```python
from build123d import *

# Parameters (mm, degrees)
F0_W        = 100
F0_H        = 50
F1_DEPTH    = 50
F2_T        = -2.5
F3_W        = 50
F3_H        = 70.2898527046
F4_DEPTH    = 25
F5_R        = 5
F6_DEPTH    = 50
F7_T1_DEPTH = 75
F7_T3_DEPTH = 75
F8_T1_DEPTH = 2.5
F8_T3_DEPTH = 2.5
F8_T5_DEPTH = 75
F9_T1_DEPTH = 75
F9_T3_DEPTH = 75
F10_R       = 11.25
F11_DEPTH   = 100


# Not quite as in the source:
# - a fillet or chamfer that OpenCascade refuses, or shapes differently, is made with other operations: its cross-section is extruded or revolved along the edge and cut away or added


with BuildPart() as f1:
    # F0 (on Top) → F1 (new body)
    with BuildSketch(Plane.XY):
        with Locations((50, 25)):
            Rectangle(F0_W, F0_H)
    extrude(amount=F1_DEPTH)

    # F2
    f2_openings = [f1.faces().sort_by_distance(p)[0] for p in [
        (50, 25, 0),
    ]]
    offset(amount=F2_T, openings=f2_openings)

    # F3 (on face) → F4 (cut)
    with BuildSketch(Plane.XY.offset(50)):
        with Locations((50, 24.9999999069)):
            Rectangle(F3_W, F3_H)
    extrude(amount=-F4_DEPTH, mode=Mode.SUBTRACT)

    # F5 (on face) → F6 (cut)
    with BuildSketch(Plane.XZ):
        with Locations((12.5, 12.5)):
            Circle(F5_R)
        with Locations((87.5, 12.5)):
            Circle(F5_R)
    extrude(amount=-F6_DEPTH, mode=Mode.SUBTRACT)

    # F7: fillet of radius 5 on 4 edges, made by hand

    # F7_s2 → F7_t1 (cut)
    with BuildSketch(Plane.XZ.offset(-62.5)):
        with BuildLine():
            ThreePointArc((0, 45), (1.4644660941, 48.5355339059), (5, 50))
            Line((5, 50), (0, 50))
            Line((0, 50), (0, 45))
        make_face()
        with BuildLine():
            ThreePointArc((0, 5), (1.4644660941, 1.4644660941), (5, 0))
            Line((5, 0), (0, 0))
            Line((0, 0), (0, 5))
        make_face()
    extrude(amount=F7_T1_DEPTH, mode=Mode.SUBTRACT)

    # F7_s4 → F7_t3 (cut)
    with BuildSketch(Plane.XY.offset(-12.5)):
        with BuildLine():
            ThreePointArc((0, 5), (1.4644660941, 1.4644660941), (5, 0))
            Line((5, 0), (0, 0))
            Line((0, 0), (0, 5))
        make_face()
        with BuildLine():
            ThreePointArc((0, 45), (1.4644660941, 48.5355339059), (5, 50))
            Line((5, 50), (0, 50))
            Line((0, 50), (0, 45))
        make_face()
    extrude(amount=F7_T3_DEPTH, mode=Mode.SUBTRACT)

    # F8: fillet of radius 5 on 6 edges, made by hand

    # F8_s2 → F8_t1 (join)
    with BuildSketch(Plane.XZ.offset(-2.5)):
        with BuildLine():
            ThreePointArc((25, 30), (26.4644660941, 26.4644660941), (30, 25))
            Line((30, 25), (25, 25))
            Line((25, 25), (25, 30))
        make_face()
        with BuildLine():
            ThreePointArc((75, 30), (73.5355339059, 26.4644660941), (70, 25))
            Line((70, 25), (75, 25))
            Line((75, 25), (75, 30))
        make_face()
    extrude(amount=F8_T1_DEPTH)

    # F8_s4 → F8_t3 (join)
    with BuildSketch(Plane.XZ.offset(-50)):
        with BuildLine():
            ThreePointArc((25, 30), (26.4644660941, 26.4644660941), (30, 25))
            Line((30, 25), (25, 25))
            Line((25, 25), (25, 30))
        make_face()
        with BuildLine():
            ThreePointArc((70, 25), (73.5355339059, 26.4644660941), (75, 30))
            Line((75, 30), (75, 25))
            Line((75, 25), (70, 25))
        make_face()
    extrude(amount=F8_T3_DEPTH)

    # F8_s6 → F8_t5 (cut)
    with BuildSketch(Plane.XZ.offset(-62.5)):
        with BuildLine():
            ThreePointArc((20, 50), (23.5355339059, 48.5355339059), (25, 45))
            Line((25, 45), (25, 50))
            Line((25, 50), (20, 50))
        make_face()
        with BuildLine():
            ThreePointArc((75, 45), (76.4644660941, 48.5355339059), (80, 50))
            Line((80, 50), (75, 50))
            Line((75, 50), (75, 45))
        make_face()
    extrude(amount=F8_T5_DEPTH, mode=Mode.SUBTRACT)

    # F9: fillet of radius 5 on 4 edges, made by hand

    # F9_s2 → F9_t1 (cut)
    with BuildSketch(Plane.XZ.offset(-62.5)):
        with BuildLine():
            ThreePointArc((100, 45), (98.5355339059, 48.5355339059), (95, 50))
            Line((95, 50), (100, 50))
            Line((100, 50), (100, 45))
        make_face()
        with BuildLine():
            ThreePointArc((95, 0), (98.5355339059, 1.4644660941), (100, 5))
            Line((100, 5), (100, 0))
            Line((100, 0), (95, 0))
        make_face()
    extrude(amount=F9_T1_DEPTH, mode=Mode.SUBTRACT)

    # F9_s4 → F9_t3 (cut)
    with BuildSketch(Plane.XY.offset(-12.5)):
        with BuildLine():
            ThreePointArc((95, 0), (98.5355339059, 1.4644660941), (100, 5))
            Line((100, 5), (100, 0))
            Line((100, 0), (95, 0))
        make_face()
        with BuildLine():
            ThreePointArc((95, 50), (98.5355339059, 48.5355339059), (100, 45))
            Line((100, 45), (100, 50))
            Line((100, 50), (95, 50))
        make_face()
    extrude(amount=F9_T3_DEPTH, mode=Mode.SUBTRACT)

    # F10 (on face) → F11 (cut)
    with BuildSketch(Plane.YZ.offset(100)):
        with Locations((25, 25.6698729811)):
            Circle(F10_R)
    extrude(amount=-F11_DEPTH, mode=Mode.SUBTRACT)


solid = f1.part
```
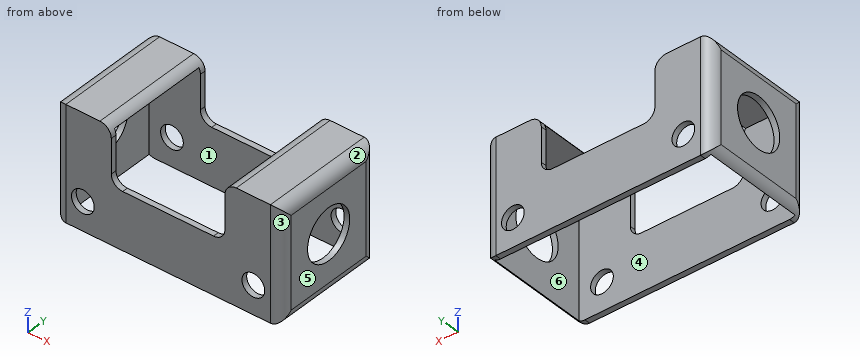
Input: part model. Units: mm. Frame: model coordinates. Face numbers are marked on the shaded views. A direction names the side the tool comes from. Round coordinates to 2 decimals unless told otherwise and drop trailing zeros. Write each loop counter-clockwise with the first axis right and the second up, starting at its lowest first coordinate (ties: lowest second). Pieces come first, ordered by that corner, then holes. Notation, with made-up numbers: (22, 86.5) - (76, 86.5) arc R21 cw to (76, 111.5) - close; hole circle Ø6 at (21, -26.5). An arc over 180 degrees is marked (long way). Write item = value, one per line.
(1) Section query D-D on y = 25. Output: boundary loops of the cut face in (x, z).
Geometry check:
outline = (0, 5) arc R5 ccw to (2.5, 0.67) - (2.5, 14.42) - (0, 14.42) - close; (0, 36.92) - (2.5, 36.92) - (2.5, 47.5) - (24.33, 47.5) arc R5 ccw to (20, 50) - (5, 50) arc R5 ccw to (0, 45) - close; (75.67, 47.5) - (97.5, 47.5) - (97.5, 36.92) - (100, 36.92) - (100, 45) arc R5 ccw to (95, 50) - (80, 50) arc R5 ccw to start; (97.5, 0.67) arc R5 ccw to (100, 5) - (100, 14.42) - (97.5, 14.42) - close
(2) Section query A-A on x = 62. Output: boundary loops of the cut face in (y, z).
Geometry check:
outline = (0, 0) - (2.5, 0) - (2.5, 25) - (0, 25) - close; (47.5, 0) - (50, 0) - (50, 25) - (47.5, 25) - close
(3) Section query B-B on y = 8. Output: boundary loops of the cut face in (x, z), then the cut area to 3 significant figures.
Geometry check:
outline = (0, 5) arc R5 ccw to (2.5, 0.67) - (2.5, 47.5) - (24.33, 47.5) arc R5 ccw to (20, 50) - (5, 50) arc R5 ccw to (0, 45) - close; (75.67, 47.5) - (97.5, 47.5) - (97.5, 0.67) arc R5 ccw to (100, 5) - (100, 45) arc R5 ccw to (95, 50) - (80, 50) arc R5 ccw to start
area = 332 mm^2
(4) Material intervals for probe 1 along Y at (x, z) = (95, 22.5); probe 2 along X at (y, z) = (37.5, 29.5); probe 3 along Z at (x, y) = (12.5, 1.9), sorted ascending.
Geometry check:
probe_1 = 0 to 2.5, 47.5 to 50
probe_2 = 0 to 2.5, 97.5 to 100
probe_3 = 0 to 7.5, 17.5 to 50
(5) Access query for the marked faces 1 and 2. Directions: +Z, -Z, +X, -X, +Y, -Y. A direction counts if a zero-diameter tool reaches every point of the face in a straight line with its end or side. Return the directions, or none.
Geometry check:
face_1 = -Z
face_2 = +Z, +X, +Y, -Y
(6) Contact query for flat-ended pins moving along their axis: pin 1 Ø1.2 at (y, z) = (0.5, 39) entering from -X; pin 2 Ø3 at (x, y) = (53.5, 49) entering from +Z; pin 3 Ø3 at (y, z) = (48.5, 34.5) entering from -X. Output: stop coordinate, or through.
Geometry check:
pin_1 = 1.87
pin_2 = 25
pin_3 = 0.42
(7) Pull-direction query (Y, two-part tool) for the marked faces 3, 4, 5 and 6; classes: +Y half, -Y half, draft (parallel to the pull), parting line (faces both ways), or undercut.
Geometry check:
face_3 = -Y half
face_4 = undercut
face_5 = draft
face_6 = undercut
(8) Section query C-C on z = 21. Output: boundary loops of the cut face in (x, y), then the cut area to 3 significant figures.
Geometry check:
outline = (0, 5) arc R5 ccw to (5, 0) - (95, 0) arc R5 ccw to (100, 5) - (100, 14.77) - (97.5, 14.77) - (97.5, 2.5) - (2.5, 2.5) - (2.5, 14.77) - (0, 14.77) - close; (0, 35.23) - (2.5, 35.23) - (2.5, 47.5) - (97.5, 47.5) - (97.5, 35.23) - (100, 35.23) - (100, 45) arc R5 ccw to (95, 50) - (5, 50) arc R5 ccw to (0, 45) - close
area = 601 mm^2
